Verification items for this drawing (mm, ordinates from the low corner). Coordinates: 2 decimals unless noted, no trailing zeros. One line per item, written item: value. Start each with the question number.
1) Scan lines: line 1 along X through (y, z) = (27.5, 2); line 2 along Y through (x, z) = (13, 0.45) (1 decimal). Record each from-to range of solid material in increasing order. Write a range as [from, to].
2) Sectioned sample at A-A on y = 29.5. Give the number of separate pieces and of enclosed holes in the cut face, plus the area to 3 significant figures.
3) Gauge pin test, flat end, axial feed: P1, Ø5.5, axis at x = 11.18, y = 28.76, coming from the -Z side. Record the tip position at first contact, or that the pin passes through.
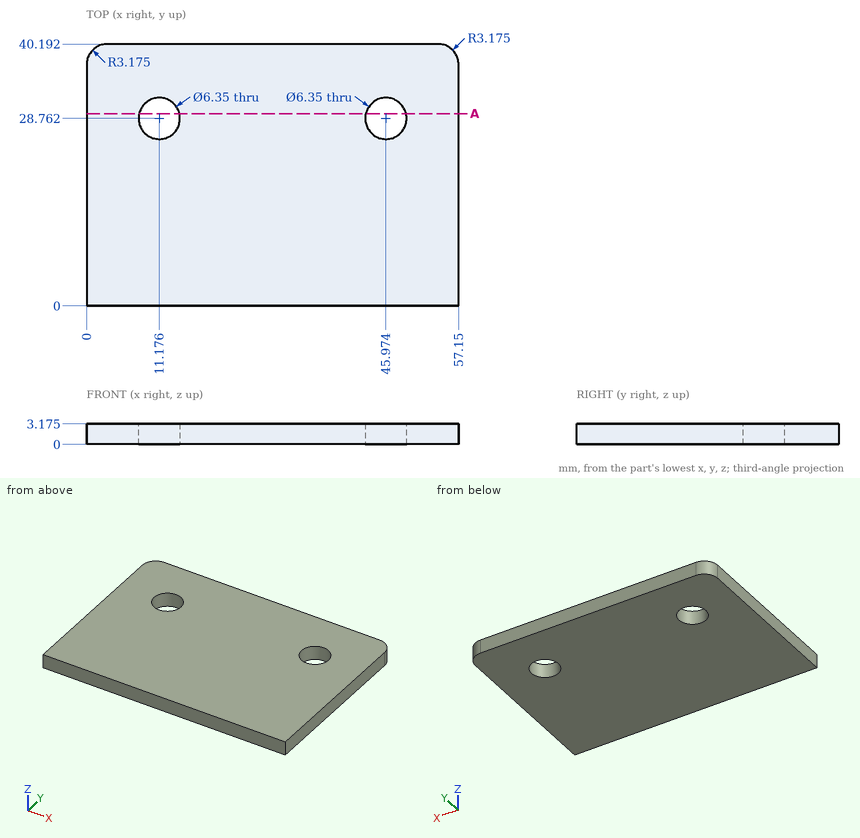
Answers:
1. line 1: x = [0, 8.26], [14.09, 43.06], [48.89, 57.15]
1. line 2: y = [0, 26.2], [31.4, 40.2]
2. separate pieces: 3
2. enclosed holes: 0
2. area: 142 mm2
3. P1: passes through
